CAD build for the part. Positions are in the model's coordinates, mm. Face numbers are marked on the shaded views. A direction names the side the tool comes from. Give positions to 0.01 mm unless a question says otherwise; leave off trailing zeros. Write each loop counter-clockwise with the first axis right and the second up, starting at its lowest first coordinate (ties: lowest second). Pieces come first, ordered by that corner, then holes. Notation, with made-up numbers: (-9.5, 5.5) -> (31.5, 5.5) arc R4 cw to (31.5, 11.5) -> close; hole circle Ø7 at (9, 60). An arc over 180 degrees is marked (long way). Answer as a JSON object with one key per item and string values.
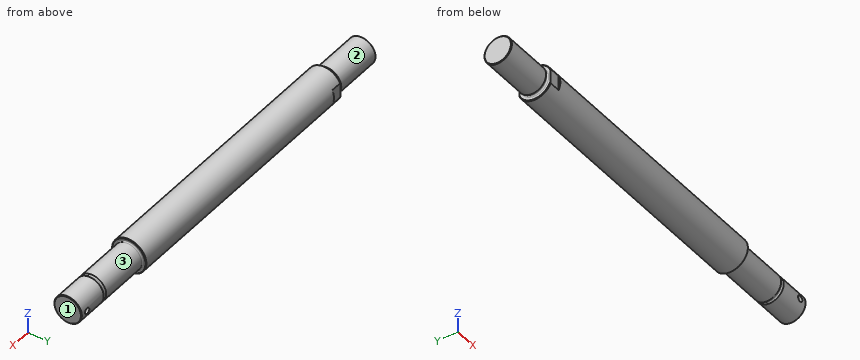
```python
from build123d import *

# Parameters (mm, degrees)
SKETCH1_W               = 356.5
SKETCH1_H               = 15
SKETCH2_W               = 3
SKETCH2_H               = 1
CUT_EXTRUDE1_DEPTH      = 180.507834091
CUT_EXTRUDE1_DEPTH_BACK = 180.507834091
SKETCH3_R               = 2.6
CUT_EXTRUDE2_DEPTH      = 180.50783419
CUT_EXTRUDE2_DEPTH_BACK = 180.50783419
SKETCH4_W               = 10
SKETCH4_H               = 1.5
FILLET1_R               = 1
CHAMFER1_SIZE           = 0.5


with BuildPart() as part:
    # Sketch1 → Revolve1 (revolve)
    with BuildSketch(Plane.XY, mode=Mode.PRIVATE) as revolve1_sk:
        with Locations((0, 7.5)):
            Rectangle(SKETCH1_W, SKETCH1_H)
    revolve(revolve1_sk.sketch.rotate(Axis((-178.25, 0, 0), (1, 0, 0)), 90), axis=Axis((-178.25, 0, 0), (1, 0, 0)))

    # Sketch2 → Cut-Revolve1 (revolve, cut)
    with BuildSketch(Plane.XY):
        Polygon((178.25, 12), (178.25, 15), (104.25, 15), (104.25, 12), (148.25, 12), (151.25, 12), align=None)
        with Locations((149.75, 11.5)):
            Rectangle(SKETCH2_W, SKETCH2_H)
        Polygon((-133.25, 15), (-178.25, 15), (-178.25, 12), (-136.25, 12), (-133.25, 12), align=None)
        with Locations((-134.75, 11.5)):
            Rectangle(SKETCH2_W, SKETCH2_H)
    revolve(axis=Axis((178.25, 0, 0), (-1, 0, 0)), mode=Mode.SUBTRACT)

    # Sketch3 → Cut-Extrude1 (cut, two sides: drawn at the far end of the back side and taken through both)
    with BuildSketch(Plane(origin=(0, 0, 0), x_dir=(1, 0, 0), z_dir=(0, 1, 0)).offset(-CUT_EXTRUDE1_DEPTH_BACK)):
        with Locations(Location((171.25, 0, 0), (0, 0, 270))):
            Circle(SKETCH3_R)
    extrude(amount=CUT_EXTRUDE1_DEPTH + CUT_EXTRUDE1_DEPTH_BACK, mode=Mode.SUBTRACT)

    # Sketch4 → Cut-Extrude2 (cut, two sides: drawn at the far end of the back side and taken through both)
    with BuildSketch(Plane.XY.offset(-CUT_EXTRUDE2_DEPTH_BACK)):
        with Locations((-128.25, 14.25)):
            Rectangle(SKETCH4_W, SKETCH4_H)
        with Locations((-128.25, -14.25)):
            Rectangle(SKETCH4_W, SKETCH4_H)
    extrude(amount=CUT_EXTRUDE2_DEPTH + CUT_EXTRUDE2_DEPTH_BACK, mode=Mode.SUBTRACT)

    # Fillet1
    fillet1_edges = [part.edges().sort_by_distance(p)[0] for p in [
        (104.25, -12, 0),
        (151.25, -11, 0),
        (148.25, -11, 0),
        (-133.25, -11, 0),
        (-136.25, -11, 0),
    ]]
    fillet(fillet1_edges, radius=FILLET1_R - 0.0001)  # a hair under: the kernel refuses the full size

    # Chamfer1
    chamfer1_edges = [part.edges().sort_by_distance(p)[0] for p in [
        (178.25, -12, 0),
        (104.25, 0, -15),
        (-178.25, -12, 0),
        (-133.25, -7.966328319, 12.709744809),
        (-133.25, 0, -15),
    ]]
    chamfer(chamfer1_edges, length=CHAMFER1_SIZE)


solid = part.part
```
1) Pin check, flat tips, straight feed: pin 1 (10 mm diameter, centred on x = 99.5, z = -7, fed in from -Y); pin 2 (5 mm diameter, centred on x = 22.5, z = -10, fed in from +Y); pin 3 (2 mm diameter, centred on x = 70, z = -1.5, fed in from -Y). Stop position of each tip, or through.
Model answer:
{"pin 1": "stops at y = -14.87", "pin 2": "stops at y = 12.99", "pin 3": "stops at y = -14.99"}
2) 3-axis set-ups, long thin cutter, end or side, ignore diameter. For the marked faces 1, 2 and 3: which of +Z, -Z, +X, -X, +Y, -Y reach the whole face in a straight line?
Model answer:
{"face 1": "+Z, -Z, +X, +Y, -Y", "face 2": "-X", "face 3": "+X"}
3) Slice it at A-A (x = 18). List the corners of the cut face in (y, z).
Model answer:
{"outline": "circle Ø30 at (0, 0)"}
4) Wall check: probe 1 along Z at (x, y) = (171.25, 3.5); probe 2 along X at (y, z) = (-4.5, 0); probe 3 along Z at (x, y) = (171.25, 0). Give the ranges that are in metal, low to high.
Model answer:
{"probe 1": "z = -11.48 to -2.6, 2.6 to 11.48", "probe 2": "x = -178.25 to 168.65, 173.85 to 178.25", "probe 3": "z = -12 to -2.6, 2.6 to 12"}
